Read the model definition and answer for the solid it produces. Units are mm, in the model's axes. Give positions to 0.01 mm unless a question says otherwise; leave off trailing zeros. Write each loop counter-clockwise with the first axis right and the second up, starting at its lowest first coordinate (ties: lowest second). Pieces come first, ordered by that corner, then holes. Notation, with made-up numbers: (30, -19) - (86, -19) arc R14 ccw to (86, -5) - close; hole circle Ø5 at (55, 43). An arc over 180 degrees is marked (long way). Answer as CSV lines item,"result".
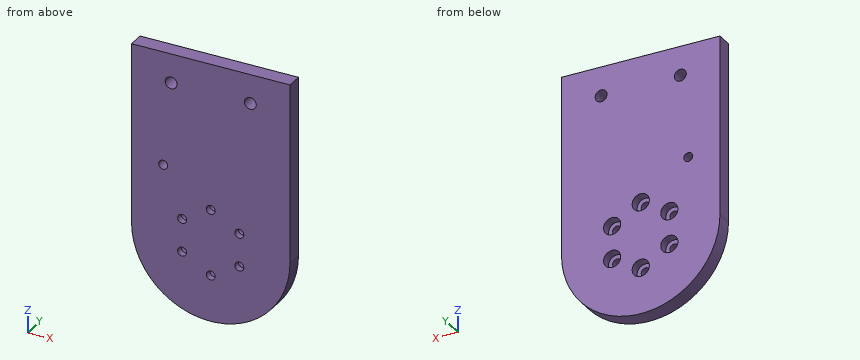
```python
from build123d import *

# Parameters (mm, degrees)
PLACA_START               = 59.75
SK_PLACA_W                = 60
SK_PLACA_H                = 49
PLACA_DEPTH               = 6
EXTREMO_START             = 59.75
SK_EXTREMO_R              = 30
EXTREMO_DEPTH             = 6
PASANTES_M3_CUBO_J3_START = 59.75
SK_PASANTES_M3_CUBO_J3_R  = 1.7
PASANTES_M3_CUBO_J3_DEPTH = 6
CAJAS_M3_J3_START         = 62.25
SK_CAJAS_M3_J3_R          = 3.25
CAJAS_M3_J3_DEPTH         = 3.5
EXTENSION_PESTANAS_START  = 59.75
SK_EXTENSION_PESTANAS_W   = 60
SK_EXTENSION_PESTANAS_H   = 19
EXTENSION_PESTANAS_DEPTH  = 6
PASANTES_M4_REPISA_START  = 59.75
SK_PASANTES_M4_REPISA_R   = 2.25
PASANTES_M4_REPISA_DEPTH  = 6
PASANTE_M3_CINCHO_START   = 59.75
SK_PASANTE_M3_CINCHO_R    = 1.7
PASANTE_M3_CINCHO_DEPTH   = 6


with BuildPart() as part:
    # Sk_Placa → Placa (new body)
    with BuildSketch(Plane(origin=(0, 0, 0), x_dir=(1, 0, 0), z_dir=(0, 1, 0)).offset(PLACA_START)):
        with Locations((0, -354.5)):
            Rectangle(SK_PLACA_W, SK_PLACA_H)
    extrude(amount=PLACA_DEPTH)

    # Sk_Extremo → Extremo (add)
    with BuildSketch(Plane(origin=(0, 0, 0), x_dir=(1, 0, 0), z_dir=(0, 1, 0)).offset(EXTREMO_START)):
        with Locations((0, -330)):
            Circle(SK_EXTREMO_R)
    extrude(amount=EXTREMO_DEPTH)

    # Sk_Pasantes_M3_cubo_J3 → Pasantes_M3_cubo_J3 (cut)
    with BuildSketch(Plane(origin=(0, 0, 0), x_dir=(1, 0, 0), z_dir=(0, 1, 0)).offset(PASANTES_M3_CUBO_J3_START)):
        with Locations(Location((10.825317547, -336.25, 0), (0, 0, 270))):
            Circle(SK_PASANTES_M3_CUBO_J3_R)
        with Locations(Location((0, -342.5, 0), (0, 0, 270))):
            Circle(SK_PASANTES_M3_CUBO_J3_R)
        with Locations(Location((-10.825317547, -336.25, 0), (0, 0, 270))):
            Circle(SK_PASANTES_M3_CUBO_J3_R)
        with Locations(Location((-10.825317547, -323.75, 0), (0, 0, 270))):
            Circle(SK_PASANTES_M3_CUBO_J3_R)
        with Locations(Location((0, -317.5, 0), (0, 0, 270))):
            Circle(SK_PASANTES_M3_CUBO_J3_R)
        with Locations(Location((10.825317547, -323.75, 0), (0, 0, 270))):
            Circle(SK_PASANTES_M3_CUBO_J3_R)
    extrude(amount=PASANTES_M3_CUBO_J3_DEPTH, mode=Mode.SUBTRACT)

    # Sk_Cajas_M3_J3 → Cajas_M3_J3 (cut)
    with BuildSketch(Plane(origin=(0, 0, 0), x_dir=(1, 0, 0), z_dir=(0, 1, 0)).offset(CAJAS_M3_J3_START)):
        with Locations(Location((10.825317547, -336.25, 0), (0, 0, 270))):
            Circle(SK_CAJAS_M3_J3_R)
        with Locations(Location((0, -342.5, 0), (0, 0, 270))):
            Circle(SK_CAJAS_M3_J3_R)
        with Locations(Location((-10.825317547, -336.25, 0), (0, 0, 270))):
            Circle(SK_CAJAS_M3_J3_R)
        with Locations(Location((-10.825317547, -323.75, 0), (0, 0, 270))):
            Circle(SK_CAJAS_M3_J3_R)
        with Locations(Location((0, -317.5, 0), (0, 0, 270))):
            Circle(SK_CAJAS_M3_J3_R)
        with Locations(Location((10.825317547, -323.75, 0), (0, 0, 270))):
            Circle(SK_CAJAS_M3_J3_R)
    extrude(amount=CAJAS_M3_J3_DEPTH, mode=Mode.SUBTRACT)

    # Sk_Extension_pestanas → Extension_pestanas (add)
    with BuildSketch(Plane(origin=(0, 0, 0), x_dir=(1, 0, 0), z_dir=(0, 1, 0)).offset(EXTENSION_PESTANAS_START)):
        with Locations((0, -388.5)):
            Rectangle(SK_EXTENSION_PESTANAS_W, SK_EXTENSION_PESTANAS_H)
    extrude(amount=EXTENSION_PESTANAS_DEPTH)

    # Sk_Pasantes_M4_repisa → Pasantes_M4_repisa (cut)
    with BuildSketch(Plane(origin=(0, 0, 0), x_dir=(1, 0, 0), z_dir=(0, 1, 0)).offset(PASANTES_M4_REPISA_START)):
        with Locations(Location((-15, -387, 0), (0, 0, 270))):
            Circle(SK_PASANTES_M4_REPISA_R)
        with Locations(Location((15, -387, 0), (0, 0, 270))):
            Circle(SK_PASANTES_M4_REPISA_R)
    extrude(amount=PASANTES_M4_REPISA_DEPTH, mode=Mode.SUBTRACT)

    # Sk_Pasante_M3_cincho → Pasante_M3_cincho (cut)
    with BuildSketch(Plane(origin=(0, 0, 0), x_dir=(1, 0, 0), z_dir=(0, 1, 0)).offset(PASANTE_M3_CINCHO_START)):
        with Locations(Location((-18, -355, 0), (0, 0, 270))):
            Circle(SK_PASANTE_M3_CINCHO_R)
    extrude(amount=PASANTE_M3_CINCHO_DEPTH, mode=Mode.SUBTRACT)


solid = part.part
```
(1) A cutting plane is placed at C-C (y = 63.4). Count the separate pieces of the cut face and the enclosed holes in it, and give its area (3 significant figures).
Worked out:
separate pieces,"1"
enclosed holes,"9"
area,"5,250 mm^2"
(2) A cutting plane is placed at B-B (x = -15). Write down the section's boundary in (y, z).
Worked out:
outline,"(59.75, 304.02) - (65.75, 304.02) - (65.75, 384.75) - (59.75, 384.75) - close; (59.75, 389.25) - (65.75, 389.25) - (65.75, 398) - (59.75, 398) - close"
(3) A cutting plane is placed at A-A (z = 336.25). Write down the section's boundary in (x, y).
Worked out:
outline,"(-30, 59.75) - (-12.53, 59.75) - (-12.53, 62.25) - (-14.08, 62.25) - (-14.08, 65.75) - (-30, 65.75) - close; (-9.13, 59.75) - (9.13, 59.75) - (9.13, 62.25) - (7.58, 62.25) - (7.58, 65.75) - (-7.58, 65.75) - (-7.58, 62.25) - (-9.13, 62.25) - close; (12.53, 59.75) - (30, 59.75) - (30, 65.75) - (14.08, 65.75) - (14.08, 62.25) - (12.53, 62.25) - close"
(4) Each of these flat-tipped pins is pushed along its axis until it touches: P1, Ø4.5, axis at x = 10.83, z = 323.75, coming from the +Y side; P2, Ø1.5, axis at y = 63, z = 314.5, coming from the -X side; P3, Ø2, axis at y = 65, z = 324.5, coming from the -X side; P4, Ø2, axis at x = 10.83, z = 336.25, coming from the +Y side. Where does it stop, or does it pass through?
Worked out:
P1,"stops at y = 62.25"
P2,"stops at x = -26.12"
P3,"stops at x = -29.66"
P4,"passes through"
(5) Find the intervals of material crossed by L1, parallel to Z at x = 11, y = 60.4; L2, parallel to Z at x = 16, y = 63.7; L3, parallel to Z at x = -14.5, y = 60.65, in increasing order.
Worked out:
L1,"z = 302.09 to 322.06, 325.44 to 334.56, 337.94 to 398"
L2,"z = 304.62 to 384.98, 389.02 to 398"
L3,"z = 303.74 to 384.81, 389.19 to 398"
(6) A cutting plane is placed at D-D (z = 317.5). Write down the section's boundary in (x, y), and give its area (3 significant figures).
Worked out:
outline,"(-27.27, 59.75) - (-1.7, 59.75) - (-1.7, 62.25) - (-3.25, 62.25) - (-3.25, 65.75) - (-27.27, 65.75) - close; (1.7, 59.75) - (27.27, 59.75) - (27.27, 65.75) - (3.25, 65.75) - (3.25, 62.25) - (1.7, 62.25) - close"
area,"296 mm^2"
